For this review, take the finished solid that the model builds, in its own axes (mm). Give positions to 0.01 mm unless a question says otherwise; leave off trailing zeros. Loops run counter-clockwise (first coordinate to the right, second up) from the corner with the lowest first, then second, coordinate; pieces in that order, holes last.
```python
from build123d import *

# Parameters (mm, degrees)
F0_W            = 80
F0_H            = 80
F1_DEPTH        = 7
F2_R            = 6
F3_DEPTH        = 5
F4_R            = 4
F5_DEPTH        = 2.001
F6_R            = 11
F6_R_2          = 1.5
F7_DEPTH        = 7.001
F8_SIZE         = 5
F10_D           = 4.4
F10_CSINK_D     = 8.96
F10_CSINK_ANGLE = 90


with BuildPart() as f1:
    # F0 (on Front) → F1 (new body)
    with BuildSketch(Plane.XZ):
        Rectangle(F0_W, F0_H)
    extrude(amount=F1_DEPTH)

    # F2 (on face) → F3 (cut)
    with BuildSketch(Plane.XZ.offset(7)):
        Circle(F2_R)
    extrude(amount=-F3_DEPTH, mode=Mode.SUBTRACT)

    # F4 (on face) → F5 (cut, through all)
    with BuildSketch(Plane.XZ.offset(2)):
        Circle(F4_R)
    extrude(amount=-F5_DEPTH, mode=Mode.SUBTRACT)

    # F6 (on face) → F7 (cut, through all)
    with BuildSketch(Plane.XZ.offset(7)):
        with Locations((-22, 0)):
            Circle(F6_R)
        with Locations((-35, 13)):
            Circle(F6_R_2)
        with Locations((-35, -13)):
            Circle(F6_R_2)
        with Locations((-9, -13)):
            Circle(F6_R_2)
        with Locations((-9, 13)):
            Circle(F6_R_2)
    extrude(amount=-F7_DEPTH, mode=Mode.SUBTRACT)

    # F8
    f8_edges = [f1.edges().sort_by_distance(p)[0] for p in [
        (-40, -3.5, 40),
        (40, -3.5, 40),
        (-40, -3.5, -40),
        (40, -3.5, -40),
    ]]
    chamfer(f8_edges, length=F8_SIZE)

    # F10 (through all)
    with Locations(Plane.XZ.offset(7)):
        with Locations((-32, 32), (32, 32), (32, -32), (-32, -32)):
            CounterSinkHole(F10_D / 2, F10_CSINK_D / 2, counter_sink_angle=F10_CSINK_ANGLE)


solid = f1.part
```
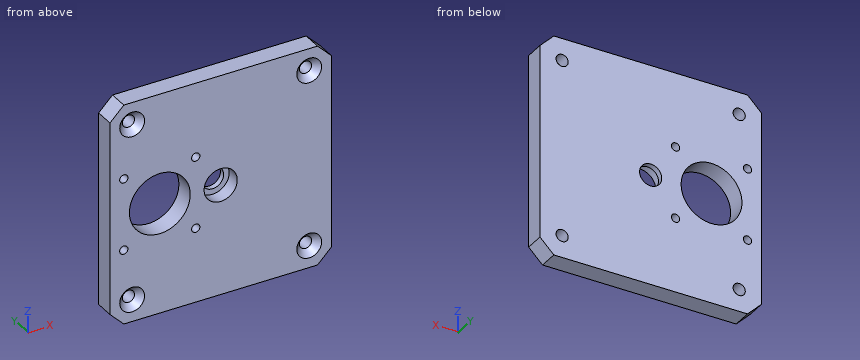
Item 1: For L1, parallel to X at y = -3, z = 32; L2, parallel to Z at x = -9, y = -3.5; L3, parallel to X at y = -0.5, z = -32.5, list the stretches that pass through material, from the lowest coordinate up.
Answer:
L1: x = -40 to -34.2, -29.8 to 29.8, 34.2 to 40
L2: z = -40 to -14.5, -11.5 to 11.5, 14.5 to 40
L3: x = -40 to -34.14, -29.86 to 29.86, 34.14 to 40
Item 2: Take a section at C-C on x = -22. Give the boundary of the cut face in (y, z), and give its area (3 significant figures).
Answer:
outline: (-7, -40) - (0, -40) - (0, -11) - (-7, -11) - close; (-7, 11) - (0, 11) - (0, 40) - (-7, 40) - close
area: 406 mm2
Item 3: Take a section at B-B on y = -3. State how many separate pieces and enclosed holes the cut face has, and give its area (3 significant figures).
Answer:
separate pieces: 1
enclosed holes: 10
area: 5,770 mm2
Item 4: Take a section at D-D on x = -9. Give the boundary of the cut face in (y, z), and give its area (3 significant figures).
Answer:
outline: (-7, -40) - (0, -40) - (0, -14.5) - (-7, -14.5) - close; (-7, -11.5) - (0, -11.5) - (0, 11.5) - (-7, 11.5) - close; (-7, 14.5) - (0, 14.5) - (0, 40) - (-7, 40) - close
area: 518 mm2
Item 5: Take a section at A-A on z = 0. Give the boundary of the cut face in (x, y), and give its area (3 significant figures).
Answer:
outline: (-40, -7) - (-33, -7) - (-33, 0) - (-40, 0) - close; (-11, -7) - (-6, -7) - (-6, -2) - (-4, -2) - (-4, 0) - (-11, 0) - close; (4, -2) - (6, -2) - (6, -7) - (40, -7) - (40, 0) - (4, 0) - close
area: 330 mm2
Item 6: Clearance check with flat-ended pins moving along their axes: pin 1 Ø5 at (x, z) = (32, -32) entering from -Y; pin 2 Ø7 at (x, z) = (-32, 32) entering from -Y; pin 3 Ø3.5 at (x, z) = (2, -2) entering from -Y. State where each tip first meets the part, or that it passes through.
Answer:
pin 1: stops at y = -5.02
pin 2: stops at y = -6.02
pin 3: stops at y = -2
